from build123d import *

# Parameters (mm, degrees)
SKETCH4_R               = 5
SKETCH4_R_2             = 1.35
BOSS_EXTRUDE1_DEPTH     = 3
SKETCH5_W               = 3
SKETCH5_H               = 40
BOSS_EXTRUDE2_DEPTH     = 60
CUT_EXTRUDE1_DEPTH      = 83.516664984
CUT_EXTRUDE1_DEPTH_BACK = 83.516664984
SKETCH7_R               = 5
SKETCH7_R_2             = 1.35
SKETCH8_R               = 5
SKETCH8_R_2             = 1.35
BOSS_EXTRUDE3_DEPTH     = 2
BOSS_EXTRUDE4_START     = -5
SKETCH10_R              = 5
SKETCH10_R_2            = 1.35
BOSS_EXTRUDE4_DEPTH     = 5
BOSS_EXTRUDE5_START     = -57
BOSS_EXTRUDE5_DEPTH     = 5


with BuildPart() as part:
    # Sketch4 → Boss-Extrude1 (new body)
    with BuildSketch(Plane(origin=(0, 0, 0), x_dir=(1, 0, 0), z_dir=(0, 1, 0))):
        Polygon((0, -20), (26.5, -20), (26.5, 20), (0, 20), (-26.5, 20), (-26.5, -20), align=None)
        with Locations(Location((0, 0, 0), (0, 0, 270))):
            Circle(SKETCH4_R, mode=Mode.SUBTRACT)
        with Locations(Location((8.012214677, 7.536870436, 0), (0, 0, 270))):
            Circle(SKETCH4_R_2, mode=Mode.SUBTRACT)
        with Locations(Location((10.994863525, -0.336119137, 0), (0, 0, 270))):
            Circle(SKETCH4_R_2, mode=Mode.SUBTRACT)
        with Locations(Location((0.336119137, 10.994863525, 0), (0, 0, 270))):
            Circle(SKETCH4_R_2, mode=Mode.SUBTRACT)
        with Locations(Location((-7.536870436, 8.012214677, 0), (0, 0, 270))):
            Circle(SKETCH4_R_2, mode=Mode.SUBTRACT)
        with Locations(Location((-10.994863525, 0.336119137, 0), (0, 0, 270))):
            Circle(SKETCH4_R_2, mode=Mode.SUBTRACT)
        with Locations(Location((-8.012214677, -7.536870436, 0), (0, 0, 270))):
            Circle(SKETCH4_R_2, mode=Mode.SUBTRACT)
        with Locations(Location((-0.336119137, -10.994863525, 0), (0, 0, 270))):
            Circle(SKETCH4_R_2, mode=Mode.SUBTRACT)
        with Locations(Location((7.536870436, -8.012214677, 0), (0, 0, 270))):
            Circle(SKETCH4_R_2, mode=Mode.SUBTRACT)
    extrude(amount=BOSS_EXTRUDE1_DEPTH)

    # Sketch5 → Boss-Extrude2 (add)
    with BuildSketch(Plane.XZ):
        with Locations((-25, 0)):
            Rectangle(SKETCH5_W, SKETCH5_H)
        with Locations((25, 0)):
            Rectangle(SKETCH5_W, SKETCH5_H)
    extrude(amount=BOSS_EXTRUDE2_DEPTH)

    # Sketch7 → Cut-Extrude1 (cut, two sides: drawn at the far end of the back side and taken through both)
    with BuildSketch(Plane(origin=(26.5, 0, 0), x_dir=(0, 0, -1), z_dir=(1, 0, 0)).offset(-CUT_EXTRUDE1_DEPTH_BACK)):
        with BuildLine():
            ThreePointArc((-10, -36.5), (-17.071067812, -33.571067812), (-20, -26.5))
            Line((-20, -26.5), (-20, -60))
            Line((-20, -60), (20, -60))
            Line((20, -60), (20, -26.5))
            ThreePointArc((20, -26.5), (17.071067812, -33.571067812), (10, -36.5))
            Line((10, -36.5), (-10, -36.5))
        make_face()
        with Locations((0, -22.5)):
            Circle(SKETCH7_R)
        with Locations((0, -11.5)):
            Circle(SKETCH7_R_2)
        with Locations((7.778174593, -14.721825407)):
            Circle(SKETCH7_R_2)
        with Locations((11, -22.5)):
            Circle(SKETCH7_R_2)
        with Locations((7.778174593, -30.278174593)):
            Circle(SKETCH7_R_2)
        with Locations((0, -33.5)):
            Circle(SKETCH7_R_2)
        with Locations((-7.778174593, -30.278174593)):
            Circle(SKETCH7_R_2)
        with Locations((-11, -22.5)):
            Circle(SKETCH7_R_2)
        with Locations((-7.778174593, -14.721825407)):
            Circle(SKETCH7_R_2)
    extrude(amount=CUT_EXTRUDE1_DEPTH + CUT_EXTRUDE1_DEPTH_BACK, mode=Mode.SUBTRACT)

    # Sketch8 → Boss-Extrude3 (add)
    with BuildSketch(Plane(origin=(0, 3, 0), x_dir=(1, 0, 0), z_dir=(0, 1, 0))):
        Polygon((-26.5, 20), (26.5, 20), (28.5, 20), (28.5, -20), (26.5, -20), (-26.5, -20), (-28.5, -20), (-28.5, 20), align=None)
        with Locations(Location((0, 0, 0), (0, 0, 270))):
            Circle(SKETCH8_R, mode=Mode.SUBTRACT)
        with Locations(Location((8.012214677, 7.536870436, 0), (0, 0, 270))):
            Circle(SKETCH8_R_2, mode=Mode.SUBTRACT)
        with Locations(Location((0.336119137, 10.994863525, 0), (0, 0, 270))):
            Circle(SKETCH8_R_2, mode=Mode.SUBTRACT)
        with Locations(Location((-7.536870436, 8.012214677, 0), (0, 0, 270))):
            Circle(SKETCH8_R_2, mode=Mode.SUBTRACT)
        with Locations(Location((-10.994863525, 0.336119137, 0), (0, 0, 270))):
            Circle(SKETCH8_R_2, mode=Mode.SUBTRACT)
        with Locations(Location((-8.012214677, -7.536870436, 0), (0, 0, 270))):
            Circle(SKETCH8_R_2, mode=Mode.SUBTRACT)
        with Locations(Location((-0.336119137, -10.994863525, 0), (0, 0, 270))):
            Circle(SKETCH8_R_2, mode=Mode.SUBTRACT)
        with Locations(Location((7.536870436, -8.012214677, 0), (0, 0, 270))):
            Circle(SKETCH8_R_2, mode=Mode.SUBTRACT)
        with Locations(Location((10.994863525, -0.336119137, 0), (0, 0, 270))):
            Circle(SKETCH8_R_2, mode=Mode.SUBTRACT)
    extrude(amount=BOSS_EXTRUDE3_DEPTH)

    # Sketch10 → Boss-Extrude4 (add)
    with BuildSketch(Plane.ZY.offset(28.5).offset(BOSS_EXTRUDE4_START)):
        with BuildLine():
            Line((-20, 3), (-20, -26.5))
            ThreePointArc((-20, -26.5), (-17.071067812, -33.571067812), (-10, -36.5))
            Line((-10, -36.5), (10, -36.5))
            ThreePointArc((10, -36.5), (17.071067812, -33.571067812), (20, -26.5))
            Line((20, -26.5), (20, 3))
            Line((20, 3), (-20, 3))
        make_face()
        with Locations(Location((0, -22.5, 0), (0, 0, 180))):
            Circle(SKETCH10_R, mode=Mode.SUBTRACT)
        with Locations(Location((-7.778174593, -14.721825407, 0), (0, 0, 180))):
            Circle(SKETCH10_R_2, mode=Mode.SUBTRACT)
        with Locations(Location((-11, -22.5, 0), (0, 0, 180))):
            Circle(SKETCH10_R_2, mode=Mode.SUBTRACT)
        with Locations(Location((-7.778174593, -30.278174593, 0), (0, 0, 180))):
            Circle(SKETCH10_R_2, mode=Mode.SUBTRACT)
        with Locations(Location((0, -33.5, 0), (0, 0, 180))):
            Circle(SKETCH10_R_2, mode=Mode.SUBTRACT)
        with Locations(Location((7.778174593, -30.278174593, 0), (0, 0, 180))):
            Circle(SKETCH10_R_2, mode=Mode.SUBTRACT)
        with Locations(Location((11, -22.5, 0), (0, 0, 180))):
            Circle(SKETCH10_R_2, mode=Mode.SUBTRACT)
        with Locations(Location((7.778174593, -14.721825407, 0), (0, 0, 180))):
            Circle(SKETCH10_R_2, mode=Mode.SUBTRACT)
        with Locations(Location((0, -11.5, 0), (0, 0, 180))):
            Circle(SKETCH10_R_2, mode=Mode.SUBTRACT)
    extrude(amount=BOSS_EXTRUDE4_DEPTH)

    # Sketch10 → Boss-Extrude5 (add)
    with BuildSketch(Plane.ZY.offset(28.5).offset(BOSS_EXTRUDE5_START)):
        with BuildLine():
            Line((-20, 3), (-20, -26.5))
            ThreePointArc((-20, -26.5), (-17.071067812, -33.571067812), (-10, -36.5))
            Line((-10, -36.5), (10, -36.5))
            ThreePointArc((10, -36.5), (17.071067812, -33.571067812), (20, -26.5))
            Line((20, -26.5), (20, 3))
            Line((20, 3), (-20, 3))
        make_face()
        with Locations(Location((0, -22.5, 0), (0, 0, 180))):
            Circle(SKETCH10_R, mode=Mode.SUBTRACT)
        with Locations(Location((-7.778174593, -14.721825407, 0), (0, 0, 180))):
            Circle(SKETCH10_R_2, mode=Mode.SUBTRACT)
        with Locations(Location((-11, -22.5, 0), (0, 0, 180))):
            Circle(SKETCH10_R_2, mode=Mode.SUBTRACT)
        with Locations(Location((-7.778174593, -30.278174593, 0), (0, 0, 180))):
            Circle(SKETCH10_R_2, mode=Mode.SUBTRACT)
        with Locations(Location((0, -33.5, 0), (0, 0, 180))):
            Circle(SKETCH10_R_2, mode=Mode.SUBTRACT)
        with Locations(Location((7.778174593, -30.278174593, 0), (0, 0, 180))):
            Circle(SKETCH10_R_2, mode=Mode.SUBTRACT)
        with Locations(Location((11, -22.5, 0), (0, 0, 180))):
            Circle(SKETCH10_R_2, mode=Mode.SUBTRACT)
        with Locations(Location((7.778174593, -14.721825407, 0), (0, 0, 180))):
            Circle(SKETCH10_R_2, mode=Mode.SUBTRACT)
        with Locations(Location((0, -11.5, 0), (0, 0, 180))):
            Circle(SKETCH10_R_2, mode=Mode.SUBTRACT)
    extrude(amount=BOSS_EXTRUDE5_DEPTH)


solid = part.part
Can you work these out from the model? Positions are in its coordinate system, mm. Coordinates: 2 decimals unless noted, no trailing zeros. Loops run counter-clockwise (first coordinate to the right, second up) from the corner with the lowest first, then second, coordinate; pieces in that order, holes last. Notation, with made-up numbers: (-8.75, 52.25) - (14.25, 52.25) arc R17 ccw to (14.25, 70.25) - close; hole circle Ø11 at (-8.75, 60.5). An arc over 180 degrees is marked (long way). Answer as a JSON object with one key per item and string values. Group by question number.
Item 1: If we section it at B-B (y = -22.5): State how many separate pieces and enclosed holes the cut face has, plus the area to 3 significant figures.
Item 2: If we section it at D-D (z = -16): List the corners of the cut face in (x, y) for me.
Item 3: If we mould it in two halves opening along Z, with no side actions, what happens to faces 1 (the face through (0, 1, 20)), 2 (the face through (-6, 0, 0)), 3 (the face through (-26.035, -22.094, -12.288)), 4 (the face through (-26.04, -33.49, -17.15))? For each: released by +Z, released by -Z, zero draft, split by the parting line, or undercut.
Item 4: If we section it at C-C (z = -11): List the corners of the cut face in (x, y) for me, plus the area to 3 significant figures.
Item 5: If I drill on L1, parallel to Y at x = 25.35, z = 0; L2, parallel to X at y = -23.5, z = -5.5; L3, parallel to Y at x = 12, z = 2, over which ranges is the centre line in solid material (lowest first)? Write a range as from..to.
Item 6: If we section it at A-A (y = -1): List the corners of the cut face in (x, z) for me.
Item 7: For pin 1 (1.5 mm diameter, centred on x = -12.5, z = 15.5, fed in from -Y), with a flat end and sliding along its axis, tell me the tip position at first contact or that it passes through.
Returned:
{
 "1": {"separate pieces": "8", "enclosed holes": "0", "area": "246 mm²"},
 "2": {"outline": "(-28.5, -34.5) - (-23.5, -34.5) - (-23.5, 0) - (23.5, 0) - (23.5, -34.5) - (28.5, -34.5) - (28.5, 5) - (-28.5, 5) - close"},
 "3": {"face 1": "released by +Z", "face 2": "zero draft", "face 3": "undercut", "face 4": "released by -Z"},
 "4": {"outline": "(-28.5, -36.45) - (-23.5, -36.45) - (-23.5, -23.85) - (-28.5, -23.85) - close; (-28.5, -21.15) - (-23.5, -21.15) - (-23.5, 0) - (-1.01, 0) - (-1.01, 5) - (-28.5, 5) - close; (1.69, 0) - (23.5, 0) - (23.5, -21.15) - (28.5, -21.15) - (28.5, 5) - (1.69, 5) - close; (23.5, -36.45) - (28.5, -36.45) - (28.5, -23.85) - (23.5, -23.85) - close", "area": "609 mm²"},
 "5": {"L1": "y = -36.5..-34.85, -32.15..-27.5, -17.5..-12.85, -10.15..5", "L2": "x = -28.5..-23.5, 23.5..28.5", "L3": "y = 0..5"},
 "6": {"outline": "(-28.5, -20) - (-23.5, -20) - (-23.5, 20) - (-28.5, 20) - close; (23.5, -20) - (28.5, -20) - (28.5, 20) - (23.5, 20) - close"},
 "7": {"pin 1": "stops at y = 0"}
}
